Design review of the part built by this model. Coordinates are the model's own, in mm. Face numbers are marked on the shaded views. A direction names the side the tool comes from. Coordinates: 2 decimals unless noted, no trailing zeros. Write each loop counter-clockwise with the first axis right and the second up, starting at its lowest first coordinate (ties: lowest second). Pieces come first, ordered by that corner, then holes.
Q1. Take a section at C-C, the plane z = 47. Write out the cut boundary in (x, y), plus the area to 3 significant figures.
Q2. Take a section at B-B, the plane x = 15.5. Write out the cut boundary in (y, z), plus the area to 3 significant figures.
Q3. Take a section at A-A, the plane y = -2.5. Write out the cut boundary in (x, z) (1 decimal).
Q4. The part is to be moulded in two halves that separate along Z. For the marked faces 1, 2, 3 and 4, say which applies: released by +Z, released by -Z, zero draft, split by the parting line, or undercut.
Q5. For the marked faces 5, 6 and 7, list the 3-axis set-ups (+Z, -Z, +X, -X, +Y, -Y) from which the entire face can be reached by the end or side of a thin tool; tool diameter is ignored.
Q6. For L1, parallel to Z at x = 7.5, y = -10; L2, parallel to Z at x = 28.5, y = -9.75; L3, parallel to X at y = -4.25, z = 7, list the stretches that pass through material, from the lowest coordinate up.
Q7. For pin 1 Ø1 at (y, z) = (-3, 18) entering from +X; pin 2 Ø1 at (x, y) = (22.5, -9.5) entering from -Z; pin 3 Ø3 at (x, y) = (41, -3.5) entering from +Z, all flat-tipped, find the tip position at first contact; note any pin that passes through.
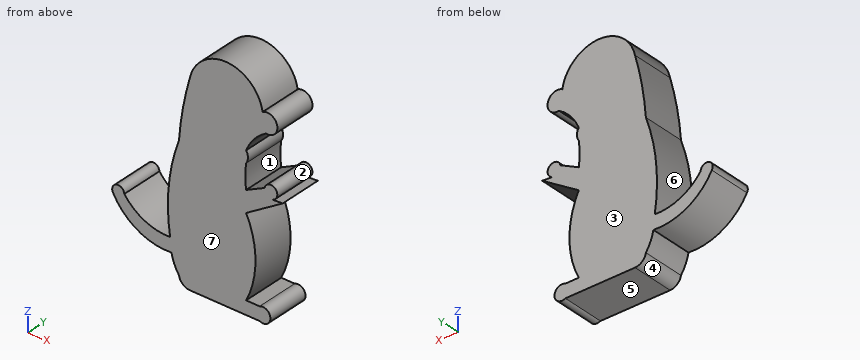
from build123d import *

# Parameters (mm, degrees)
F1_DEPTH = 12.7


with BuildPart() as f1:
    # F0 (on Front) → F1 (new body)
    with BuildSketch(Plane.XZ):
        with BuildLine():
            ThreePointArc((45.659669, 43.789603), (49.07354, 47.207987), (44.703573, 49.267903))
            ThreePointArc((44.703573, 49.267903), (34.051612, 58.522614), (22.955889, 49.804881))
            ThreePointArc((22.955889, 49.804881), (20.871145, 40.757723), (19.714734, 31.545777))
            ThreePointArc((19.714734, 31.545777), (16.650538, 17.976794), (17.055664, 4.072029))
            ThreePointArc((17.055664, 4.072029), (9.415581, 5.443728), (3.358493, 10.298016))
            ThreePointArc((3.358493, 10.298016), (1.016335, 11.924756), (0, 9.260352))
            ThreePointArc((0, 9.260352), (7.346914, 2.010702), (17.47073, 0))
            ThreePointArc((17.47073, 0), (18.301019, -2.776931), (19.714734, -5.307176))
            ThreePointArc((19.714734, -5.307176), (20.827914, -7.282535), (22.955889, -8.06544))
            Line((22.955889, -8.06544), (39.524082, -8.06544))
            Line((39.524082, -8.06544), (43.786854, -8.06544))
            ThreePointArc((43.786854, -8.06544), (47.032645, -6.05943), (43.786854, -4.053419))
            Line((43.786854, -4.053419), (39.774835, -4.053419))
            ThreePointArc((39.774835, -4.053419), (42.573385, 7.857265), (39.774835, 19.767949))
            Line((39.774835, 19.767949), (50.701622, 26.749119))
            Line((50.701622, 26.749119), (47.29737, 26.538234))
            ThreePointArc((47.29737, 26.538234), (48.612442, 29.727127), (45.29136, 28.794995))
            Line((45.29136, 28.794995), (39.774835, 26.03673))
            ThreePointArc((39.774835, 26.03673), (39.482213, 29.672624), (39.774835, 33.308517))
            ThreePointArc((39.774835, 33.308517), (40.316203, 35.063775), (39.774835, 36.819033))
            ThreePointArc((39.774835, 36.819033), (42.127254, 40.802418), (45.659669, 43.789603))
        make_face()
    extrude(amount=F1_DEPTH)


solid = f1.part
Responses:
1. outline: (22.21, -12.7) - (49.1, -12.7) - (49.1, 0) - (22.21, 0) - close
1. area: 342 mm2
2. outline: (-12.7, -0.08) - (0, -0.08) - (0, 4.04) - (-12.7, 4.04) - close
2. area: 52.3 mm2
3. outline: (0, 9.3) arc R18 ccw to (17.5, 0) arc R13.3 ccw to (19.7, -5.3) arc R3.3 ccw to (23, -8.1) - (43.8, -8.1) arc R2.2 ccw (long way) to (43.8, -4.1) - (39.8, -4.1) arc R26.7 ccw to (39.8, 19.8) - (50.7, 26.7) - (47.3, 26.5) arc R1.9 ccw (long way) to (45.3, 28.8) - (39.8, 26) arc R22.7 cw to (39.8, 33.3) arc R3.1 ccw to (39.8, 36.8) arc R13.9 cw to (45.7, 43.8) arc R3 ccw (long way) to (44.7, 49.3) arc R11.1 ccw to (23, 49.8) arc R91.4 ccw to (19.7, 31.5) arc R55.5 ccw to (17.1, 4.1) arc R15.8 cw to (3.4, 10.3) arc R1.8 ccw (long way) to start
4. face 1: undercut
4. face 2: undercut
4. face 3: zero draft
4. face 4: released by -Z
5. face 5: -Z, -X, +Y, -Y
5. face 6: +Y, -Y
5. face 7: +Z, -Z, +X, -X, -Y
6. L1: z = 1.93 to 6.48
6. L2: z = -8.07 to 57.19
6. L3: x = 1.47 to 6.73, 16.68 to 42.56
7. pin 1: stops at x = 40.77
7. pin 2: stops at z = -8.07
7. pin 3: stops at z = 56.93
